```python
from build123d import *

# Parameters (mm, degrees)
SKETCH1_R               = 40
SKETCH1_R_2             = 25
BOSS_EXTRUDE1_DEPTH     = 50
SKETCH2_R               = 40
SKETCH2_R_2             = 37.5
BOSS_EXTRUDE2_DEPTH     = 5
SKETCH3_R               = 1
CUT_EXTRUDE2_DEPTH      = 41
CUT_EXTRUDE2_DEPTH_BACK = 41
SKETCH4_W               = 1
SKETCH4_H               = 6.6
CUT_EXTRUDE3_DEPTH      = 41.0000001
CIRPATTERN1_COUNT       = 4
CIRPATTERN1_ANGLE       = 135
SKETCH5_R               = 61.08994387
CUT_EXTRUDE4_DEPTH      = 2.6


with BuildPart() as part:
    # Sketch1 → Boss-Extrude1 (new body)
    with BuildSketch(Plane(origin=(0, 0, 0), x_dir=(1, 0, 0), z_dir=(0, 1, 0))):
        Circle(SKETCH1_R)
        Circle(SKETCH1_R_2, mode=Mode.SUBTRACT)
    extrude(amount=BOSS_EXTRUDE1_DEPTH)

    # Sketch2 → Boss-Extrude2 (add)
    with BuildSketch(Plane.XZ):
        Circle(SKETCH2_R)
        Circle(SKETCH2_R_2, mode=Mode.SUBTRACT)
    extrude(amount=BOSS_EXTRUDE2_DEPTH)

    # Sketch3 → Cut-Extrude2 (cut, two sides)
    with BuildSketch(Plane(origin=(0, 0, 0), x_dir=(0, 0, -1), z_dir=(1, 0, 0))) as cut_extrude2_sk:
        with Locations((0, 30.95)):
            Circle(SKETCH3_R)
    extrude(amount=CUT_EXTRUDE2_DEPTH, mode=Mode.SUBTRACT)
    extrude(cut_extrude2_sk.sketch, amount=-CUT_EXTRUDE2_DEPTH_BACK, mode=Mode.SUBTRACT)

    # Sketch4 → Cut-Extrude3 (cut, symmetric)
    with BuildSketch(Plane.XY):
        with Locations((0, -1.7)):
            Rectangle(SKETCH4_W, SKETCH4_H)
    cut_extrude3 = extrude(amount=CUT_EXTRUDE3_DEPTH, both=True, mode=Mode.SUBTRACT)

    # CirPattern1: Cut-Extrude3 ×4 about axis
    cirpattern1_axis = Axis((0, 0, 0), (0, 1, 0))
    for i in range(1, CIRPATTERN1_COUNT):
        add(cut_extrude3.rotate(cirpattern1_axis, i * CIRPATTERN1_ANGLE / (CIRPATTERN1_COUNT - 1)), mode=Mode.SUBTRACT)

    # Sketch5 → Cut-Extrude4 (cut)
    with BuildSketch(Plane.XZ.offset(5)):
        Circle(SKETCH5_R)
    extrude(amount=-CUT_EXTRUDE4_DEPTH, mode=Mode.SUBTRACT)


solid = part.part
```
Verification items for the finished model (mm, model axes). A direction names the side the tool comes from. Coordinates: 2 decimals unless noted, no trailing zeros. Loops run counter-clockwise (first coordinate to the right, second up) from the corner with the lowest first, then second, coordinate; pieces in that order, holes last. Notation, with made-up numbers: (11.25, -3.5) - (53.25, -3.5) arc R20 cw to (53.25, 16.5) - close; hole circle Ø9 at (7.25, 60.25). An arc over 180 degrees is marked (long way). Put each result on its own line as item: value.
Item 1: Section check A-A (x = 7). Enter the section's corners in (y, z), then the cut area to 3 significant figures.
Conclusion:
outline: (-2.4, -39.38) - (50, -39.38) - (50, -24) - (0, -24) - (0, -36.84) - (-2.4, -36.84) - close; (-2.4, 36.84) - (0, 36.84) - (0, 24) - (50, 24) - (50, 39.38) - (-2.4, 39.38) - close
area: 1,550 mm2
Item 2: Gauge pin test, flat ends, axial feed: pin 1 Ø0.5 at (x, z) = (0, 31) entering from -Y; pin 2 Ø1.2 at (x, y) = (32, -1.5) entering from -Z; pin 3 Ø3.5 at (x, z) = (23.5, 23.5) entering from -Y; pin 4 Ø1.6 at (y, z) = (30.95, 0) entering from +X. Record the tip position at first contact, or that the pin passes through.
Conclusion:
pin 1: stops at y = 1.6
pin 2: stops at z = -24.78
pin 3: stops at y = 0
pin 4: passes through
Item 3: Section check B-B (z = -13). Enter the section's corners in (x, y), then the cut area to 3 significant figures.
Conclusion:
outline: (-37.83, -2.4) - (-35.17, -2.4) - (-35.17, 0) - (-21.35, 0) - (-21.35, 50) - (-37.83, 50) - close; (21.35, 0) - (35.17, 0) - (35.17, -2.4) - (37.83, -2.4) - (37.83, 50) - (21.35, 50) - close
area: 1,660 mm2
Item 4: Section check D-D (x = 33). Enter the section's corners in (y, z).
Conclusion:
outline: (-2.4, -22.61) - (50, -22.61) - (50, 22.61) - (-2.4, 22.61) - (-2.4, 17.81) - (0, 17.81) - (0, 0.5) - (1.6, 0.5) - (1.6, -0.5) - (0, -0.5) - (0, -17.81) - (-2.4, -17.81) - close; hole circle Ø2 at (30.95, 0)
Item 5: Draft check along Z on faces 1 (the face through (-34.57, -1.18, 14.53)), 2 (the face through (34.3, 0.5, 0.5)), 3 (the face through (-8.67, 24.17, -39.05)), 4 (the face through (14, -2.4, 35)). Enter one of: pulls with the +Z half, pulls with the -Z half, needs draft (parallel to the pull), parting line crosses it, or undercut.
Conclusion:
face 1: undercut
face 2: undercut
face 3: parting line crosses it
face 4: needs draft
Item 6: Set-up check for faces 5 (the face through (0.5, 0.5, 34.3)), 6 (the face through (-28, 0, -14)), 7 (the face through (34.3, 0.5, -0.5)): record each of +Z, -Z, +X, -X, +Y, -Y from which the full face is reachable in a straight line by a thin tool's end or side.
Conclusion:
face 5: +Z, -Z, -Y
face 6: -Y
face 7: +X, -X, -Y
Item 7: Scan lines: line 1 along Z through (x, y) = (0, 27); line 2 along Y through (x, z) = (34.5, 0); line 3 along Y through (x, z) = (-12.5, -24.5). Record each from-to range of solid material in increasing order.
Conclusion:
line 1: z = -40 to -25, 25 to 40
line 2: y = 1.6 to 29.95, 31.95 to 50
line 3: y = 0 to 50
